```python
from build123d import *

# Parameters (mm, degrees)
SKETCH1_W           = 87.3125
SKETCH1_H           = 34.925
BOSS_EXTRUDE1_DEPTH = 3.175
CUT_EXTRUDE2_DEPTH  = 48.126295158


with BuildPart() as part:
    # Sketch1 → Boss-Extrude1 (new body)
    with BuildSketch(Plane(origin=(0, 0, 0), x_dir=(1, 0, 0), z_dir=(0, 1, 0))):
        Rectangle(SKETCH1_W, SKETCH1_H)
    extrude(amount=BOSS_EXTRUDE1_DEPTH)

    # Sketch3 → Cut-Extrude2 (cut, through all)
    with BuildSketch(Plane.XZ):
        Polygon((-26.8732, 17.4625), (-23.9268, 17.4625), (-23.9268, 13.462), (-22.987, 13.462), (-22.987, 11.811), (-23.9268, 11.811), (-23.9268, 7.8105), (-26.8732, 7.8105), (-26.8732, 11.811), (-27.813, 11.811), (-27.813, 13.462), (-26.8732, 13.462), align=None)
        Polygon((26.8732, 11.811), (26.8732, 7.8105), (23.9268, 7.8105), (23.9268, 11.811), (22.987, 11.811), (22.987, 13.462), (23.9268, 13.462), (23.9268, 17.4625), (26.8732, 17.4625), (26.8732, 13.462), (27.813, 13.462), (27.813, 11.811), align=None)
        Polygon((26.8732, -17.4625), (23.9268, -17.4625), (23.9268, -13.462), (22.987, -13.462), (22.987, -11.811), (23.9268, -11.811), (23.9268, -7.8105), (26.8732, -7.8105), (26.8732, -11.811), (27.813, -11.811), (27.813, -13.462), (26.8732, -13.462), align=None)
        Polygon((-26.8732, -11.811), (-26.8732, -7.8105), (-23.9268, -7.8105), (-23.9268, -11.811), (-22.987, -11.811), (-22.987, -13.462), (-23.9268, -13.462), (-23.9268, -17.4625), (-26.8732, -17.4625), (-26.8732, -13.462), (-27.813, -13.462), (-27.813, -11.811), align=None)
    extrude(amount=-CUT_EXTRUDE2_DEPTH, mode=Mode.SUBTRACT)


solid = part.part
```
Input: part model. Units: mm. Frame: model coordinates. A direction names the side the tool comes from. Round coordinates to 2 decimals unless told otherwise and drop trailing zeros. Loops run counter-clockwise (first coordinate to the right, second up) from the corner with the lowest first, then second, coordinate; pieces in that order, holes last. Notation, with made-up numbers: (36.5, 2) - (79.5, 2) arc R20 cw to (79.5, 6) - close; hole circle Ø4 at (13, 65.5). An arc over 180 degrees is marked (long way). One line per item, written item: value. Start each with the question number.
(1) Ray query, line 1 (X direction, y = 0.75, z = 8.5); line 2 (Z direction, x = 23.5, y = 0.6); line 3 (X direction, y = 2.65, z = -13). Return the intervals inside material, ascending. Write a range as [from, to].
(2) Section A-A, the plane z = 9. Return loops of the section in (x, y) (3 decimals), plus the area to 3 significant figures.
(3) Access query for faces 4 (the flat face through (25, 2, 7.81)), 5 (the flat face through (27.813, 2, -13)), 6 (the flat face through (35, 2, 17.462)), 7 (the flat face through (23.927, 2, -15)). Directions: +Z, -Z, +X, -X, +Y, -Y. A direction counts if a zero-diameter tool reaches every point of the face in a straight line with its end or side. Return the directions, or none.
(4) Draft query along X for faces 1 (the flat face through (23.927, 2, -10)), 2 (the flat face through (35, 2, -17.462)), 3 (the flat face through (-43.656, 2, 0)). Return one class per face: +X half, -X half, draft (parallel to the pull), parting line (faces both ways), or undercut.
Results below:
1. line 1: [-43.66, -26.87], [-23.93, 23.93], [26.87, 43.66]
1. line 2: [-17.46, -13.46], [-11.81, 11.81], [13.46, 17.46]
1. line 3: [-43.66, -27.81], [-22.99, 22.99], [27.81, 43.66]
2. outline: (-43.656, 0) - (-26.873, 0) - (-26.873, 3.175) - (-43.656, 3.175) - close; (-23.927, 0) - (23.927, 0) - (23.927, 3.175) - (-23.927, 3.175) - close; (26.873, 0) - (43.656, 0) - (43.656, 3.175) - (26.873, 3.175) - close
2. area: 259 mm^2
3. face 4: +Z, +Y, -Y
3. face 5: +Y, -Y
3. face 6: +Z, +X, -X, +Y, -Y
3. face 7: -Z, +Y, -Y
4. face 1: undercut
4. face 2: draft
4. face 3: -X half
